from build123d import *

# Parameters (mm, degrees)
SKETCH1_R           = 9.15
BOSS_EXTRUDE1_DEPTH = 65
SKETCH2_R           = 2.5
CUT_EXTRUDE1_DEPTH  = 10
CHAMFER1_SIZE2      = 0.25
CHAMFER1_SIZE       = 10
CUT_EXTRUDE2_START  = -10
SKETCH3_R           = 2.5
CUT_EXTRUDE2_DEPTH  = 10
CHAMFER2_SIZE2      = 0.25
CHAMFER2_SIZE       = 10


with BuildPart() as part:
    # Sketch1 → Boss-Extrude1 (new body)
    with BuildSketch(Plane(origin=(0, 0, 0), x_dir=(1, 0, 0), z_dir=(0, 1, 0))):
        with Locations(Location((0, 0, 0), (0, 0, 270))):
            Circle(SKETCH1_R)
    extrude(amount=BOSS_EXTRUDE1_DEPTH)

    # Sketch2 → Cut-Extrude1 (cut)
    with BuildSketch(Plane(origin=(0, 65, 0), x_dir=(1, 0, 0), z_dir=(0, 1, 0))):
        with Locations(Location((0, 0, 0), (0, 0, 270))):
            Circle(SKETCH2_R)
    extrude(amount=-CUT_EXTRUDE1_DEPTH, mode=Mode.SUBTRACT)

    # Chamfer1
    chamfer1_edges = [part.edges().sort_by_distance(p)[0] for p in [
        (0, 55, -2.5),
    ]]
    chamfer1_side = [part.faces().sort_by_distance(p)[0] for p in [
        (0, 55.005, -2.5),
    ]]
    chamfer(chamfer1_edges, length=CHAMFER1_SIZE - 0.0001, length2=CHAMFER1_SIZE2 - 0.0001, reference=chamfer1_side[0])  # a hair under: the kernel refuses the full size

    # Sketch3 → Cut-Extrude2 (cut)
    with BuildSketch(Plane.XZ.offset(CUT_EXTRUDE2_START)):
        with Locations(Location((0, 0, 0), (0, 0, 270))):
            Circle(SKETCH3_R)
    extrude(amount=CUT_EXTRUDE2_DEPTH, mode=Mode.SUBTRACT)

    # Chamfer2
    chamfer2_edges = [part.edges().sort_by_distance(p)[0] for p in [
        (0, 10, 2.5),
    ]]
    chamfer2_side = [part.faces().sort_by_distance(p)[0] for p in [
        (0, 9.995, 2.5),
    ]]
    chamfer(chamfer2_edges, length=CHAMFER2_SIZE - 0.0001, length2=CHAMFER2_SIZE2 - 0.0001, reference=chamfer2_side[0])  # a hair under: the kernel refuses the full size


solid = part.part
Could you check a few things on this model? Use its own coordinates, in mm. A direction names the side the tool comes from. Round coordinates to 2 decimals unless told otherwise and drop trailing zeros. Order: outer loops, then holes, each group sorted by start corner. A loop starts at its lowest first (then second) coordinate and runs counter-clockwise, first axis right, second up.
Q1. Imagine slicing it at D-D, the plane x = -8. List the corners of the cut face in (y, z) for me, then the cut area to 3 significant figures.
Geometry says:
outline: (0, -4.44) - (65, -4.44) - (65, 4.44) - (0, 4.44) - close
area: 577 mm2
Q2. Please list where these lines run through material, in increasing order: probe 1 along X at (y, z) = (0.05, 0); probe 2 along Y at (x, z) = (1.25, -1.25); probe 3 along Z at (x, y) = (-0.25, 33.5).
Geometry says:
probe 1: x = -9.15 to -2.5, 2.5 to 9.15
probe 2: y = 10 to 55
probe 3: z = -9.15 to 9.15
Q3. I'm going to push flat-ended pins straight in: P1, Ø2, axis at x = 7.5, y = 58, coming from the +Z side; P2, Ø6, axis at y = 54.5, z = -5, coming from the +X side; P3, Ø10, axis at x = 6, y = 56.5, coming from the -Z side. Where does each tip first touch, or does it pass through?
Geometry says:
P1: stops at z = 6.44
P2: stops at x = 8.93
P3: stops at z = -9.1
Q4. Thinking about a two-plate mould opening in X: for faces 1 (the face through (2.748, 32.045, 8.727)), 2 (the face through (0, 10, 0)), 3 (the face through (-2, 65, 2)), which applies, released by +X, released by -X, zero draft, split by the parting line, or undercut?
Geometry says:
face 1: split by the parting line
face 2: undercut
face 3: zero draft
Q5. Imagine slicing it at C-C, the plane y = 51.5. List the corners of the cut face in (x, z) for me, then the cut area to 3 significant figures.
Geometry says:
outline: circle Ø18.3 at (0, 0)
area: 263 mm2
Q6. Which directions (+Z, -Z, +X, -X, +Y, -Y) give clear straight access to the entire face, cutting with the end or side of a thin tool? Please do faces 4 (the face through (0.713, 59.93, 2.264)), 5 (the face through (0.713, 5.07, -2.264)), 6 (the face through (-2, 0, 2)).
Geometry says:
face 4: +Y
face 5: -Y
face 6: +Z, -Z, +X, -X, -Y
